Could you check a few things on this model? Use its own coordinates, in mm. Face numbers are marked on the shaded views. A direction names the side the tool comes from. Give positions to 0.01 mm unless a question says otherwise; leave off trailing zeros. Write each loop counter-clockwise with the first axis right and the second up, starting at its lowest first coordinate (ties: lowest second). Pieces come first, ordered by that corner, then holes. Notation, with made-up numbers: M -24,0.25 L 14,0.25 A18 cw 14,21.25 Z; hole C 75,-9 d11. An arc over 180 degrees is marked long. One line per item, written item: value.
```python
from build123d import *

# Parameters (mm, degrees)
HEX_CUT_DEPTH = 1.1


with BuildPart() as part:
    # Body_Sketch → Body_Revolve (revolve)
    with BuildSketch(Plane(origin=(0, 0, 0), x_dir=(0, 0, -1), z_dir=(1, 0, 0)), mode=Mode.PRIVATE) as body_revolve_sk:
        Polygon((0, 1.5), (10.04, 1.5), (10.14, 1.4), (10.14, 0), (-1.86, 0), (-1.86, 2.675), (-1.175, 2.675), align=None)
    revolve(body_revolve_sk.sketch.rotate(Axis((0, 0, 0), (0, 0, -1)), 90), axis=Axis((0, 0, 0), (0, 0, -1)))

    # Key_Sketch → Hex_Cut (cut)
    with BuildSketch(Plane.XY.offset(1.86)):
        Polygon((1.154700538, 0), (0.577350269, 1), (-0.577350269, 1), (-1.154700538, 0), (-0.577350269, -1), (0.577350269, -1), align=None)
    extrude(amount=-HEX_CUT_DEPTH, mode=Mode.SUBTRACT)


solid = part.part
```
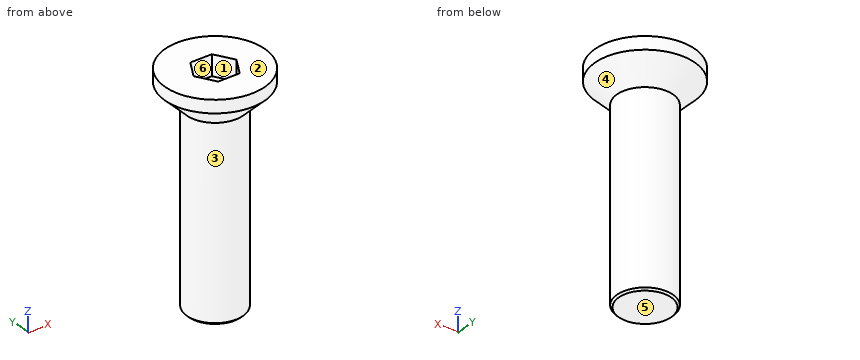
1) If we section it at A-A, the plane x = 0: Write out the boundary of the cut face in (y, z) (3 decimals), then the cut area to 3 significant figures.
Outcome:
outline: M -2.675,1.175 L -1.5,0 L -1.5,-10.04 L -1.4,-10.14 L 1.4,-10.14 L 1.5,-10.04 L 1.5,0 L 2.675,1.175 L 2.675,1.86 L 1,1.86 L 1,0.76 L -1,0.76 L -1,1.86 L -2.675,1.86 Z
area: 36.8 mm^2
2) On a 3-axis mill with a long thin cutter (end or side, diameter ignored), from which of +Z, -Z, +X, -X, +Y, -Y can I reach the whole of each face in a straight line? I mean the marked faces 1, 2 and 3. Say none if no direction works.
Outcome:
face 1: +Z
face 2: +Z, +X, -X, +Y, -Y
face 3: -Z
3) Please list where these lines run through material, in increasing order: L1, parallel to X at y = -2, z = 1; L2, parallel to Z at x = -1.4, y = -1.4; L3, parallel to X at y = 0.75, z = -1.5. Write a range as from..to.
Outcome:
L1: x = -1.5..1.5
L2: z = 0.48..1.86
L3: x = -1.3..1.3
4) We'd pull the mould along X, two halves only. Please class the marked faces 4, 5 and 6: pulls with the +X half, pulls with the -X half, needs draft (parallel to the pull), parting line crosses it, or undercut.
Outcome:
face 4: parting line crosses it
face 5: needs draft
face 6: undercut
5) I'm going to push flat-ended pins straight in: pin 1 (1.5 mm diameter, centred on y = -1, z = -6.5, fed in from -X); pin 2 (0.6 mm diameter, centred on x = 0, y = 0.5, fed in from +Z); pin 3 (2 mm diameter, centred on x = -1, z = 0, fed in from +Y). Where does each tip first touch, or does it pass through?
Outcome:
pin 1: stops at x = -1.48
pin 2: stops at z = 0.76
pin 3: stops at y = 2.35
6) If we section it at B-B, the plane z = -1.5: Write out the boundary of the cut face in (x, y).
Outcome:
outline: C 0,0 d3
